Build history of the part. All positions in model axes, mm. Coordinates: 2 decimals unless noted, no trailing zeros. Loops run counter-clockwise (first coordinate to the right, second up) from the corner with the lowest first, then second, coordinate; pieces in that order, holes last.
Item 1: Drill centre lines: line 1 along Y through (x, z) = (173.6, 178); line 2 along Y through (x, z) = (171.25, 191); line 3 along Y through (x, z) = (169.75, 256). Where is each one in solid material? Low to high.
Item 2: Cut at A-A (z = 237). List the corners of the cut face in (x, y), and give its area (3 significant figures).
Item 3: Cut at B-B (x = 173.5). List the corners of the cut face in (y, z), and give its area (3 significant figures).
Item 4: Cut at D-D (y = 188). List the corners of the cut face in (x, z).
Item 5: Cut at C-C (z = 226). List the corners of the cut face in (x, y), and give its area (3 significant figures).
Item 6: Mould opens along Y. For faces 1 (the face through (176, 114, 268)), 2 (the face through (170.93, 112.611, 276.975)), 3 (the face through (170.93, 112.831, 266.978)) say: released by +Y, released by -Y, zero draft, split by the parting line, or undercut.
Item 7: Flat gauge pins, fed straight in: pin 1 (1 mm diameter, centred on x = 170, y = 166, fed in from -Z); pin 2 (1.5 mm diameter, centred on x = 168.5, y = 161, fed in from +Z); pin 3 (2 mm diameter, centred on y = 6, z = 178, fed in from +X); pin 4 (3 mm diameter, centred on y = 6.5, z = 178, fed in from +X). Where does each tip first touch, or does it go through?
from build123d import *

# Parameters (mm, degrees)
BOX105_W          = 202
BOX105_H          = 239
BOX105_DEPTH      = 10
CYLINDER080_R     = 1.3
CYLINDER080_DEPTH = 331
CYLINDER078_R     = 1.3
CYLINDER078_DEPTH = 331
CYLINDER079_W     = 105
CYLINDER079_H     = 10
CYLINDER079_ANGLE = 180
CYLINDER077_W     = 115
CYLINDER077_H     = 10
CYLINDER077_ANGLE = 180


with BuildPart() as cubo068:
    # Box105 → Box105 (new body)
    with BuildSketch(Plane.XY.offset(162)):
        with Locations((101, 119.5)):
            Rectangle(BOX105_W, BOX105_H)
    extrude(amount=BOX105_DEPTH)


with BuildPart() as cilindro080:
    # Cylinder080 → Cylinder080 (new body)
    with BuildSketch(Plane(origin=(5, 224, 178), x_dir=(0, 0, -1), z_dir=(1, 0, 0))):
        Circle(CYLINDER080_R)
    extrude(amount=CYLINDER080_DEPTH)


with BuildPart() as cilindro078:
    # Cylinder078 → Cylinder078 (new body)
    with BuildSketch(Plane(origin=(5, 6, 178), x_dir=(0, 0, -1), z_dir=(1, 0, 0))):
        Circle(CYLINDER078_R)
    extrude(amount=CYLINDER078_DEPTH)


with BuildPart() as cilindro079:
    # Cylinder079 → Cylinder079 (revolve)
    with BuildSketch(Plane(origin=(-3, 115, 171), x_dir=(0, -1, 0), z_dir=(0, 0, -1))):
        with Locations((52.5, 5)):
            Rectangle(CYLINDER079_W, CYLINDER079_H)
    revolve(axis=Axis((-3, 115, 171), (-1, 0, 0)), revolution_arc=CYLINDER079_ANGLE)


with BuildPart() as cut091:
    # Cylinder077 → Cylinder077 (revolve)
    with BuildSketch(Plane(origin=(-3, 115, 171), x_dir=(0, -1, 0), z_dir=(0, 0, -1))):
        with Locations((57.5, 5)):
            Rectangle(CYLINDER077_W, CYLINDER077_H)
    revolve(axis=Axis((-3, 115, 171), (-1, 0, 0)), revolution_arc=CYLINDER077_ANGLE)

    # Cut086: cut Cilindro079
    add(cilindro079.part, mode=Mode.SUBTRACT)


with BuildPart() as cut091_1:
    # Cut086 placement: moved
    add(cut091.part.moved(Location((13, 0, -9))))

    # Cut087: cut Cilindro078
    add(cilindro078.part, mode=Mode.SUBTRACT)

    # Cut085: cut Cilindro080
    add(cilindro080.part, mode=Mode.SUBTRACT)


with BuildPart() as cut091_2:
    # Cut085 placement: moved
    add(cut091_1.part.moved(Location((166, 0, 0))))

    # Cut091: cut Cubo068
    add(cubo068.part, mode=Mode.SUBTRACT)


solid = cut091_2.part
Filled sheet:
1. line 1: y = 1.12 to 4.7, 7.3 to 11.23, 218.77 to 222.7, 225.3 to 228.88
1. line 2: y = 3.72 to 14.08, 215.92 to 226.28
1. line 3: y = 48.75 to 68.21, 161.79 to 181.25
2. outline: (166, 27.82) - (176, 27.82) - (176, 41.52) - (166, 41.52) - close; (166, 188.48) - (176, 188.48) - (176, 202.18) - (166, 202.18) - close
2. area: 274 mm2
3. outline: (0.44, 172) - (10.48, 172) arc R105 cw to (219.52, 172) - (229.56, 172) arc R115 ccw to start; hole circle Ø2.6 at (6, 178); hole circle Ø2.6 at (224, 178)
3. area: 3,240 mm2
4. outline: (166, 237.47) - (176, 237.47) - (176, 250.86) - (166, 250.86) - close
5. outline: (166, 19.45) - (176, 19.45) - (176, 31.76) - (166, 31.76) - close; (166, 198.24) - (176, 198.24) - (176, 210.55) - (166, 210.55) - close
5. area: 246 mm2
6. face 1: zero draft
6. face 2: split by the parting line
6. face 3: undercut
7. pin 1: stops at z = 253.5
7. pin 2: stops at z = 267.72
7. pin 3: stops at x = 171
7. pin 4: stops at x = 176
